```python
from build123d import *
from OCP.BRepFilletAPI import BRepFilletAPI_MakeChamfer

# Parameters (mm, degrees)
SKETCH1_R           = 7.5
BOSS_EXTRUDE1_DEPTH = 89.838116
SKETCH2_R           = 4.298993134
CUT_EXTRUDE1_DEPTH  = 91.462075404
CHAMFER1_SIZE       = 1.784416
CHAMFER1_SIZE2      = 1.030233


with BuildPart() as part:
    # Sketch1 → Boss-Extrude1 (new body)
    with BuildSketch(Plane(origin=(0, 0, 0), x_dir=(1, 0, 0), z_dir=(0, 1, 0))):
        with Locations(Location((0, 0, 0), (0, 0, 270))):
            Circle(SKETCH1_R)
    extrude(amount=BOSS_EXTRUDE1_DEPTH)

    # Sketch2 → Cut-Extrude1 (cut, through all)
    with BuildSketch(Plane(origin=(0, 0, 0), x_dir=(1, 0, 0), z_dir=(0, 1, 0))):
        with Locations(Location((0, 0, 0), (0, 0, 270))):
            Circle(SKETCH2_R)
    extrude(amount=CUT_EXTRUDE1_DEPTH, mode=Mode.SUBTRACT)

    # Chamfer1: one chamfer whose edges measure the first distance from different faces: ONE call of the kernel's chamfer builder (chamfer() names one face for all edges)
    chamfer1_edges_1 = [part.edges().sort_by_distance(p)[0] for p in [
        (0, 0, -7.5),
    ]]
    chamfer1_side_1 = [part.faces().sort_by_distance(p)[0] for p in [
        (0, 0, -7.287867966),
    ]]
    chamfer1_edges_2 = [part.edges().sort_by_distance(p)[0] for p in [
        (0, 89.838116, -7.5),
    ]]
    chamfer1_side_2 = [part.faces().sort_by_distance(p)[0] for p in [
        (0, 44.919058, -7.5),
    ]]
    chamfer1 = BRepFilletAPI_MakeChamfer(part.part.solid().wrapped)
    for e in chamfer1_edges_1:
        chamfer1.Add(CHAMFER1_SIZE, CHAMFER1_SIZE2, e.wrapped, chamfer1_side_1[0].wrapped)  # the first distance lies on this face
    for e in chamfer1_edges_2:
        chamfer1.Add(CHAMFER1_SIZE, CHAMFER1_SIZE2, e.wrapped, chamfer1_side_2[0].wrapped)  # the first distance lies on this face
    add(Compound.cast(chamfer1.Shape()), mode=Mode.REPLACE)


solid = part.part
```
Geometry check sheet. Reference: the model listing, model coordinates, mm. Coordinates: 2 decimals unless noted, no trailing zeros. Write each loop counter-clockwise with the first axis right and the second up, starting at its lowest first coordinate (ties: lowest second). Pieces come first, ordered by that corner, then holes. Notation, with made-up numbers: M 26.5,61.5 L 63.5,61.5 A14 ccw 63.5,77.5 Z; hole C -11,18.5 d9. An arc over 180 degrees is marked long. One line per item, written item: value. Start each with the question number.
(1) Sectioned sample at C-C, the plane y = 12. Enter the section's corners in (x, z), and give its area (3 significant figures).
(2) Sectioned sample at A-A, the plane z = 0. Enter the section's corners in (x, y).
(3) Sectioned sample at B-B, the plane x = 0. Enter the section's corners in (y, z), and give its area (3 significant figures).
(4) Scan lines: line 1 along X through (y, z) = (42.5, 0); line 2 along X through (y, z) = (67, 1.5); line 3 along Z through (x, y) = (0.5, 63). Record each from-to range of solid material in increasing order. Write a range as [from, to].
(5) Release check for a two-part mould opening along Z. For faces 1 (the face through (0.33, 43.933, -7.493)), 2 (the face through (1.29, 44.29, 4.1)), 3 (the face through (4, 0, -2)) record: released by +Z, released by -Z, zero draft, split by the parting line, or undercut.
(6) Depth check by flat-ended pin: pin 1 (5 mm diameter, centred on y = 37, z = 5.5, fed in from -X); pin 2 (7 mm diameter, centred on x = 0, z = 0, fed in from +Y) (3 decimals); pin 3 (1.5 mm diameter, centred on y = 14.5, z = 1, fed in from -X); pin 4 (1 mm diameter, centred on x = 5.5, z = -3.5, fed in from -Y). Enter the tip coordinate at first touch or a pass-through.
Filled sheet:
1. outline: C 0,0 d15; hole C 0,0 d8.6
1. area: 119 mm²
2. outline: M -7.5,1.03 L -5.72,0 L -4.3,0 L -4.3,89.84 L -6.47,89.84 L -7.5,88.05 Z; M 4.3,0 L 5.72,0 L 7.5,1.03 L 7.5,88.05 L 6.47,89.84 L 4.3,89.84 Z
3. outline: M 0,-5.72 L 1.03,-7.5 L 88.05,-7.5 L 89.84,-6.47 L 89.84,-4.3 L 0,-4.3 Z; M 0,4.3 L 89.84,4.3 L 89.84,6.47 L 88.05,7.5 L 1.03,7.5 L 0,5.72 Z
3. area: 571 mm²
4. line 1: [-7.5, -4.3], [4.3, 7.5]
4. line 2: [-7.35, -4.03], [4.03, 7.35]
4. line 3: [-7.48, -4.27], [4.27, 7.48]
5. face 1: split by the parting line
5. face 2: undercut
5. face 3: zero draft
6. pin 1: x = -6.87
6. pin 2: through
6. pin 3: x = -7.5
6. pin 4: y = 0.18
